Could you check a few things on this model? Use its own coordinates, in mm. A direction names the side the tool comes from. Give positions to 0.01 mm unless a question says otherwise; leave off trailing zeros. Order: outer loops, then holes, each group sorted by start corner. A loop starts at its lowest first (then second) coordinate and runs counter-clockwise, first axis right, second up. Notation, with made-up numbers: (27, -2.75) -> (63, -2.75) arc R20 ccw to (63, 30.25) -> close; hole circle Ø6 at (11.5, 20.25). An arc over 180 degrees is marked (long way). One line per item, written item: value.
```python
from build123d import *

# Parameters (mm, degrees)
F0_W     = 965.2
F0_H     = 965.2
F1_DEPTH = 482.6
F2_W     = 685.8
F2_H     = 685.8
F3_DEPTH = 965.201
F5_DEPTH = 279.4
F7_DEPTH = 279.4
F9_DEPTH = 50.8


with BuildPart() as f1:
    # F0 (on Top) → F1 (new body, symmetric)
    with BuildSketch(Plane.XY):
        Rectangle(F0_W, F0_H)
    extrude(amount=F1_DEPTH, both=True)

    # F2 (on face) → F3 (cut, through all)
    with BuildSketch(Plane(origin=(-482.6, 0, 0), x_dir=(0, -1, 0), z_dir=(-1, 0, 0))):
        with Locations((139.7, 139.7)):
            Rectangle(F2_W, F2_H)
    extrude(amount=-F3_DEPTH, mode=Mode.SUBTRACT)

    # F4 (on face) → F5 (join, through all)
    with BuildSketch(Plane.XZ.offset(-203.2)):
        with BuildLine():
            Line((-482.6, 482.6), (482.6, 482.6))
            ThreePointArc((482.6, 482.6), (0, 965.2), (-482.6, 482.6))
        make_face()
    extrude(amount=-F5_DEPTH)

    # F6 (on face) → F7 (join, through all)
    with BuildSketch(Plane.XY.offset(-203.2)):
        with BuildLine():
            Line((482.6, -482.6), (-482.6, -482.6))
            ThreePointArc((-482.6, -482.6), (0, -965.2), (482.6, -482.6))
        make_face()
    extrude(amount=-F7_DEPTH)

    # F8 (on Right) → F9 (join, symmetric)
    with BuildSketch(Plane.YZ):
        Polygon((-762, -203.2), (203.2, -203.2), (203.2, 762), align=None)
    extrude(amount=F9_DEPTH, both=True)


solid = f1.part
```
1) Suppose I cut it at A-A, the plane z = 161. Write out the boundary of the cut face in (x, y).
Answer below:
outline: (-482.6, 203.2) -> (-50.8, 203.2) -> (-50.8, -397.8) -> (50.8, -397.8) -> (50.8, 203.2) -> (482.6, 203.2) -> (482.6, 482.6) -> (-482.6, 482.6) -> close
2) For P1, Ø2, axis at y = 76.5, z = 386, coming from the +X side; P2, Ø1, axis at x = -372, y = 245.5, coming from the +Z side; P3, Ø12, axis at x = 294.5, z = 70.5, coming from the -Y side, each with a flat end and sliding along its axis, tell me the tip position at first contact or that it passes through.
Answer below:
P1: stops at x = 50.8
P2: stops at z = 790.64
P3: stops at y = 203.2
3) Suppose I cut it at D-D, the plane z = -376. Write out the boundary of the cut face in (x, y).
Answer below:
outline: (-482.6, -482.6) arc R482.6 ccw to (482.6, -482.6) -> (482.6, 482.6) -> (-482.6, 482.6) -> close
4) Suppose I cut it at B-B, the plane y = -348. Write out the boundary of the cut face in (x, z), then the cut area to 3 significant figures.
Answer below:
outline: (-482.6, -482.6) -> (482.6, -482.6) -> (482.6, -203.2) -> (50.8, -203.2) -> (50.8, 210.8) -> (-50.8, 210.8) -> (-50.8, -203.2) -> (-482.6, -203.2) -> close
area: 312,000 mm2
5) If I drill on line 1 along Z through (x, y) = (-123.5, 161); line 2 along Y through (x, z) = (-106, 128); line 3 along X through (y, z) = (82, -87.5), over which ranges is the centre line in solid material (lowest first)?
Answer below:
line 1: z = -482.6 to -203.2
line 2: y = 203.2 to 482.6
line 3: x = -50.8 to 50.8
6) For faces 1 (the flat face through (-50.8, -72, 72)), 2 (the flat face through (-114, 203.2, 389)), 3 (the flat face through (482.6, 208, -100)), 4 (the flat face through (50.8, -72, 72)), which set-ups out of +Z, -Z, +X, -X, +Y, -Y let a thin tool reach every point of the face, with its end or its side?
Answer below:
face 1: +Z, -X, -Y
face 2: +Z, -Y
face 3: +Z, -Z, +X, +Y, -Y
face 4: +Z, +X, -Y
7) Suppose I cut it at C-C, the plane x = 0. Write out the boundary of the cut face in (y, z).
Answer below:
outline: (-965.2, -482.6) -> (482.6, -482.6) -> (482.6, 965.2) -> (203.2, 965.2) -> (203.2, 762) -> (-762, -203.2) -> (-965.2, -203.2) -> close
